from build123d import *

# Parameters (mm, degrees)
EXTRUDE_1_DEPTH     = 10
EXTRUDE_2_DEPTH     = 10
SKETCH_5_W          = 3.14
SKETCH_5_H          = 5.14
CUT_EXTRUDE_1_DEPTH = 3
SCALE_1_SCALE       = 1.5


with BuildPart() as part:
    # 스케치2 → 보스-돌출1 (new body)
    with BuildSketch(Plane(origin=(0, 0, 0), x_dir=(1, 0, 0), z_dir=(0, 1, 0))):
        Polygon((8.485281374, -8.485281374), (0, 0), (-8.485281374, -8.485281374), (-12.727922061, -8.485281374), (0, 4.242640687), (12.727922061, -8.485281374), align=None)
    extrude(amount=EXTRUDE_1_DEPTH)

    # 스케치3 → 보스-돌출2 (add)
    with BuildSketch(Plane(origin=(0, 10, 0), x_dir=(1, 0, 0), z_dir=(0, 1, 0))):
        Polygon((-6.949747468, -2.707106781), (-2, 2.242640687), (-6.949747468, 2.242640687), align=None)
        Polygon((2, 2.242640687), (6.949747468, -2.707106781), (6.949747468, 2.242640687), align=None)
    extrude(amount=-EXTRUDE_2_DEPTH)

    # 스케치5 → 컷-돌출1 (cut)
    with BuildSketch(Plane(origin=(0, 0, -2.242640687), x_dir=(-1, 0, 0), z_dir=(0, 0, -1))):
        with Locations((-4.57, 5)):
            Rectangle(SKETCH_5_W, SKETCH_5_H)
        with Locations((4.57, 5)):
            Rectangle(SKETCH_5_W, SKETCH_5_H)
    extrude(amount=-CUT_EXTRUDE_1_DEPTH, mode=Mode.SUBTRACT)


with BuildPart() as part_1:
    # 축척1: scaled about (0, 5, 2.601544192)
    add(part.part.scale(SCALE_1_SCALE).moved(Location((0, -2.5, -1.300772096))))


solid = part_1.part
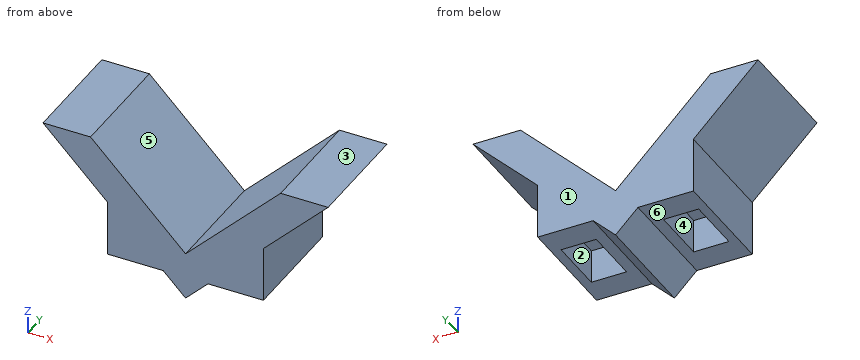
Model file for the job. Use its own axes, mm. Face numbers are marked on the shaded views. A direction names the side the tool comes from. Round coordinates to 2 decimals unless told otherwise and drop trailing zeros. Order: outer loops, then holes, each group sorted by start corner. A loop starts at its lowest first (then second) coordinate and runs counter-clockwise, first axis right, second up. Notation, with made-up numbers: M -10.5,25.25 L -6.5,25.25 A10 ccw -6.5,38.25 Z; hole C 34,-6.5 d5. An arc over 180 degrees is marked long. Write each question's results on one line, items separated by ' | '. Start each with the question number.
(1) Saw through at D-D, the plane y = 6. Give the cut face in (x, z).
(2) Probe probe 1 along X at (y, z) = (5.25, -3.25); probe 2 along Y at (x, z) = (-6, -4) (3 decimals); probe 3 along X at (y, z) = (4, 3.75). List the from-to ranges inside material, lowest first. Write a range as from..to.
(3) Drop flat-ended pins along their axis: pin 1 (1.4 mm diameter, centred on x = 7, y = 5, fed in from -Z); pin 2 (8 mm diameter, centred on y = 3, z = -0.5, fed in from -X); pin 3 (8 mm diameter, centred on y = 2.5, z = -2, fed in from +X); pin 4 (5 mm diameter, centred on x = -11, z = -1, fed in from +Y). Give the stop position or say it passes through.
(4) Saw through at C-C, the plane x = -6. Give the cut face in (y, z) (3 decimals), then the cut area to 3 significant figures.
(5) Saw through at B-B, the plane z = 0.75. Give the cut face in (x, y).
(6) Which spindle directions (+Z, -Z, +X, -X, +Y, -Y) get a long thin tool onto all of the face, cutting with end or side? Do the marked faces 4, 5 and 6. Say none if no direction does.
(7) Saw through at A-A, the plane y = -0.5. Give the cut face in (x, z), then the cut area to 3 significant figures.
(8) Two-plate mould, pull along Y, no slides. Class the marked faces 1, 2 and 3: pulls with the +Y half, pulls with the -Y half, needs draft (parallel to the pull), parting line crosses it, or undercut.
Established:
1) outline: M -19.09,11.43 L -10.42,2.76 L -10.42,-4.66 L -9.21,-4.66 L -9.21,-0.16 L -4.5,-0.16 L -4.5,-4.66 L -3,-4.66 L 0,-7.66 L 3,-4.66 L 4.5,-4.66 L 4.5,-0.16 L 9.21,-0.16 L 9.21,-4.66 L 10.42,-4.66 L 10.42,2.76 L 19.09,11.43 L 12.73,11.43 L 0,-1.3 L -12.73,11.43 Z
2) probe 1: x = -10.42..-9.21, -4.5..4.5, 9.21..10.42 | probe 2: y = -2.5..1.145, 8.855..12.5 | probe 3: x = -11.41..-5.05, 5.05..11.41
3) pin 1: stops at z = -0.16 | pin 2: stops at x = -11.16 | pin 3: stops at x = 10.42 | pin 4: stops at y = 12.5
4) outline: M -2.5,-4.665 L 1.145,-4.665 L 1.145,-0.165 L 8.855,-0.165 L 8.855,-4.665 L 12.5,-4.665 L 12.5,4.699 L -2.5,4.699 Z | area: 106 mm^2
5) outline: M -10.42,-2.5 L -2.05,-2.5 L -2.05,12.5 L -10.42,12.5 Z; M 2.05,-2.5 L 10.42,-2.5 L 10.42,12.5 L 2.05,12.5 Z
6) face 4: -Z | face 5: +Z, +Y, -Y | face 6: -Z, -X, +Y, -Y
7) outline: M -19.09,11.43 L -10.42,2.76 L -10.42,-4.66 L -3,-4.66 L 0,-7.66 L 3,-4.66 L 10.42,-4.66 L 10.42,2.76 L 19.09,11.43 L 12.73,11.43 L 0,-1.3 L -12.73,11.43 Z | area: 258 mm^2
8) face 1: pulls with the +Y half | face 2: undercut | face 3: needs draft
